Drawing for the job (mm, zero at the part's lowest x, y, z). Give positions to 0.01 mm unless a question says otherwise; leave off trailing zeros. Write each loop counter-clockwise with the first axis right and the second up, starting at its lowest first coordinate (ties: lowest second). Pieces come first, ordered by that corner, then holes. Notation, with made-up numbers: M 86.5,44 L 107.5,44 A33 cw 107.5,77 Z; hole C 50.5,60.25 d9. An arc over 180 degrees is marked long. Write item = value, one per line. Start each with the question number.
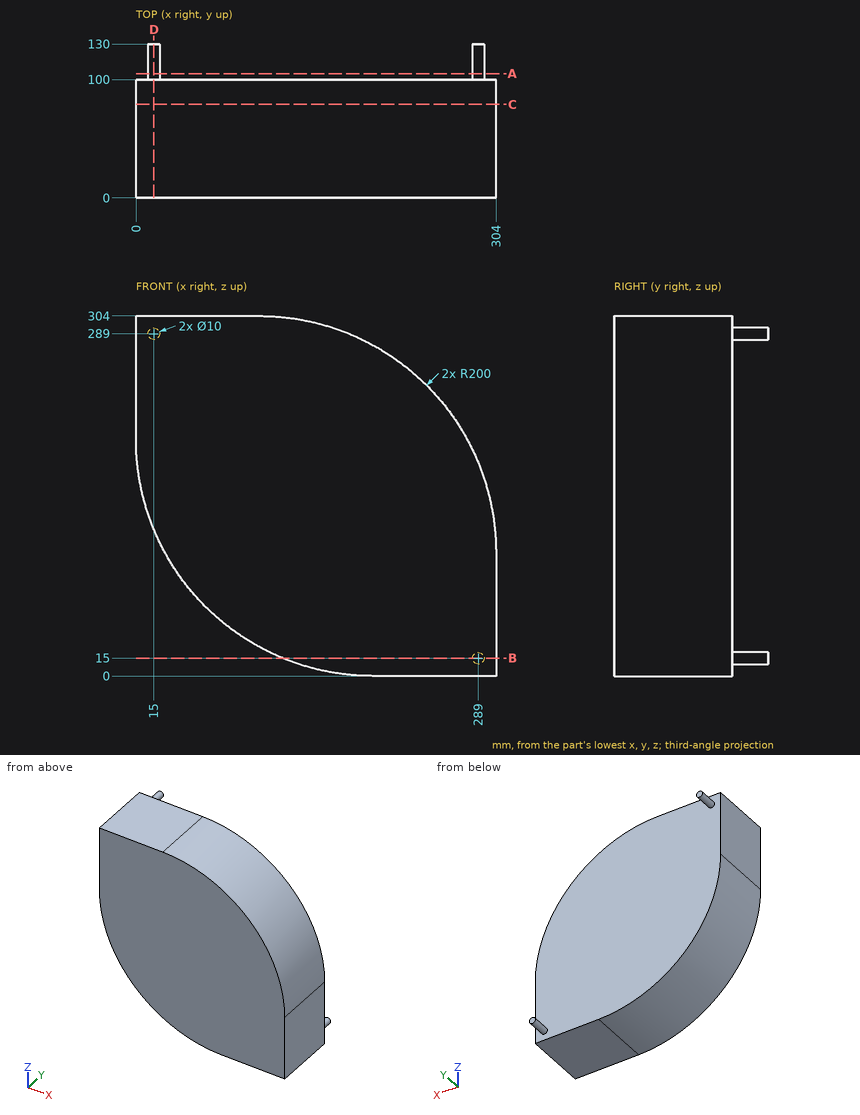
Q1. Probe line 1 along Y through (x, z) = (164, 185); line 2 along Z through (x, y) = (67.5, 22); line 3 along X through (y, z) = (60.5, 246). List the from-to ranges inside material, lowest first.
Q2. Drop flat-ended pins along their axis: P1, Ø12, axis at x = 230, z = 125.5, coming from the +Y side; P2, Ø1.5, axis at x = 271, y = 102, coming from the +Z side; P3, Ø8, axis at y = 77.5, z = 173.5, coming from the +X side; P4, Ø4, axis at y = 101.5, z = 116.5, coming from the -X side. Give the stop position or say it passes through.
Q3. Slice it at B-B (z = 15). Give the cut face in (x, y), and give its area (3 significant figures).
Q4. Slice it at D-D (x = 15). Give the cut face in (y, z), and give its area (3 significant figures).
Q5. Slice it at C-C (y = 79). Give the cut face in (x, z), and give its area (3 significant figures).
Q6. Slice it at A-A (y = 105). Give the cut face in (x, z), and give its area (3 significant figures).
Working result:
q1.line_1 = 0 to 100
q1.line_2 = 50.19 to 304
q1.line_3 = 0 to 244.84
q2.P1 = 100
q2.P2 = through
q2.P3 = 292.97
q2.P4 = 17.66
q3.outline = M 124.01,0 L 304,0 L 304,100 L 294,100 L 294,130 L 284,130 L 284,100 L 124.01,100 Z
q3.area = 18,300 mm2
q4.outline = M 0,124.01 L 100,124.01 L 100,284 L 130,284 L 130,294 L 100,294 L 100,304 L 0,304 Z
q4.area = 18,300 mm2
q5.outline = M 0,200 A200 ccw 200,0 L 304,0 L 304,104 A200 ccw 104,304 L 0,304 Z
q5.area = 75,200 mm2
q6.outline = C 15,289 d10; C 289,15 d10
q6.area = 157 mm2
